```python
from build123d import *

# Parameters (mm, degrees)
BOSS_EXTRUDE1_DEPTH = 4.826
SKETCH4_R           = 6.35
CUT_EXTRUDE5_DEPTH  = 5.826


with BuildPart() as part:
    # Sketch1 → Boss-Extrude1 (new body)
    with BuildSketch(Plane.XY):
        Polygon((-26.67, -22.21179672), (30.48, -22.21179672), (45.271508428, 32.990864252), (-41.461508428, 32.990864252), align=None)
    extrude(amount=BOSS_EXTRUDE1_DEPTH)

    # Sketch4 → Cut-Extrude5 (cut, through all)
    with BuildSketch(Plane.XY):
        with Locations((0, 5.389533766)):
            Circle(SKETCH4_R)
    extrude(amount=CUT_EXTRUDE5_DEPTH, mode=Mode.SUBTRACT)


solid = part.part
```
Design review of the part built by this model. Coordinates are the model's own, in mm. Coordinates: 2 decimals unless noted, no trailing zeros. Order: outer loops, then holes, each group sorted by start corner. A loop starts at its lowest first (then second) coordinate and runs counter-clockwise, first axis right, second up. Notation, with made-up numbers: (18, -3) - (48, -3) arc R28 ccw to (48, 27) - close; hole circle Ø3 at (-37.5, 44.5). An arc over 180 degrees is marked (long way). Answer in a Markdown table with one row per item.
(1) Consider section B-B on y = 7. State the section outline as (x, z) points, plus the area to 3 significant figures.
Checked values:
| item | result |
|---|---|
| outline | (-34.5, 0) - (-6.14, 0) - (-6.14, 4.83) - (-34.5, 4.83) - close; (6.14, 0) - (38.31, 0) - (38.31, 4.83) - (6.14, 4.83) - close |
| area | 292 mm^2 |
(2) Wall thickness on line 1 along Y through (x, z) = (0, 1.4); line 2 along Y through (x, z) = (-5, 0.3); line 3 along X through (y, z) = (10, 3.4): over which ranges is each line inside the solid? List them lowest first. Write a range as from..to.
Checked values:
| item | result |
|---|---|
| line 1 | -22.21..-0.96, 11.74..32.99 |
| line 2 | -22.21..1.48, 9.3..32.99 |
| line 3 | -35.3..-4.37, 4.37..39.11 |
(3) Consider section C-C on z = 3.95. State the section outline as (x, y) points.
Checked values:
| item | result |
|---|---|
| outline | (-41.46, 32.99) - (-26.67, -22.21) - (30.48, -22.21) - (45.27, 32.99) - close; hole circle Ø12.7 at (0, 5.39) |
(4) Consider section D-D on x = -32. State the section outline as (y, z) points, plus the area to 3 significant figures.
Checked values:
| item | result |
|---|---|
| outline | (-2.32, 0) - (32.99, 0) - (32.99, 4.83) - (-2.32, 4.83) - close |
| area | 170 mm^2 |
(5) The part is to be moulded in two halves that separate along X. For faces 1 (the cylindrical face through (-1.38, -0.81, 2.38)), 2 (the flat face through (1, 12, 0)), 3 (the flat face through (37.77, 5, 2.38)), say which applies: released by +X, released by -X, zero draft, split by the parting line, or undercut.
Checked values:
| item | result |
|---|---|
| face 1 | undercut |
| face 2 | zero draft |
| face 3 | released by +X |
(6) Consider section A-A on x = 0. State the section outline as (y, z) points.
Checked values:
| item | result |
|---|---|
| outline | (-22.21, 0) - (-0.96, 0) - (-0.96, 4.83) - (-22.21, 4.83) - close; (11.74, 0) - (32.99, 0) - (32.99, 4.83) - (11.74, 4.83) - close |
